from build123d import *

# Parameters (mm, degrees)
F0_R     = 25.4
F1_DEPTH = 12.7
F2_R     = 12.7
F3_DEPTH = 25.4
F4_R     = 2.54
F4_R_2   = 6.35
F5_DEPTH = 25.4


with BuildPart() as f1:
    # F0 (on Top) → F1 (new body)
    with BuildSketch(Plane.XY):
        Circle(F0_R)
    extrude(amount=F1_DEPTH)

    # F2 (on Top) → F3 (join)
    with BuildSketch(Plane.XY):
        Circle(F2_R)
    extrude(amount=F3_DEPTH)

    # F4 (on Top) → F5 (cut)
    with BuildSketch(Plane.XY):
        with Locations((0, 19.05)):
            Circle(F4_R)
        with Locations((-19.05, 0)):
            Circle(F4_R)
        with Locations((0, -19.05)):
            Circle(F4_R)
        with Locations((19.05, 0)):
            Circle(F4_R)
        Circle(F4_R_2)
    extrude(amount=F5_DEPTH, mode=Mode.SUBTRACT)


solid = f1.part
Source: CAD feature listing. Evaluate the final solid. Frame: model axes, mm. Give positions to 0.01 mm unless a question says otherwise; leave off trailing zeros. Write each loop counter-clockwise with the first axis right and the second up, starting at its lowest first coordinate (ties: lowest second). Pieces come first, ordered by that corner, then holes. Notation, with made-up numbers: M -11,25 L 8,25 A33 cw 8,53 Z; hole C 33.5,12 d2. An arc over 180 degrees is marked long. Return JSON: item names as keys, results as strings. Group by question number.
1) Cut plane D-D, the plane z = 20.75. Output: boundary loops of the cut face in (x, y), plus the area to 3 significant figures.
2) Cut plane C-C, the plane x = -19.05. Output: boundary loops of the cut face in (y, z), plus the area to 3 significant figures.
3) Pull-direction query (Y, two-part tool) for faces 1 (the face through (-0.33, -16.53, 6.26)), 2 (the face through (-12, -5, 12.7)), 3 (the face through (-2.75, -12.4, 18.96)); classes: pulls with the +Y half, pulls with the -Y half, needs draft (parallel to the pull), parting line crosses it, or undercut.
4) Pin query (flat end, axial travel): P1, Ø3, axis at y = -1.5, z = 8.5, coming from the +X side; P2, Ø7.5, axis at x = 0, y = 0, coming from the -Z side; P3, Ø1.5, axis at y = 8, z = 11, coming from the -X side; P4, Ø5, axis at x = 4, z = 13.5, coming from the -Y side. Return the tip coordinate at first contact, or that it passes through.
5) Cut plane A-A, the plane x = 0. Output: boundary loops of the cut face in (y, z).
6) Material intervals for line 1 along Y through (x, z) = (0, 9); line 2 along Z through (x, y) = (-9, -17.5); line 3 along X through (y, z) = (19.05, 10.25), sorted ascending. Write a range as [from, to].
7) Cut plane B-B, the plane y = 5. Output: boundary loops of the cut face in (x, z).
Recorded:
{
 "1": {"outline": "C 0,0 d25.4; hole C 0,0 d12.7", "area": "380 mm²"},
 "2": {"outline": "M -16.8,0 L -2.54,0 L -2.54,12.7 L -16.8,12.7 Z; M 2.54,0 L 16.8,0 L 16.8,12.7 L 2.54,12.7 Z", "area": "362 mm²"},
 "3": {"face 1": "undercut", "face 2": "needs draft", "face 3": "parting line crosses it"},
 "4": {"P1": "stops at x = 25.4", "P2": "passes through", "P3": "stops at x = -24.34", "P4": "stops at y = -25.35"},
 "5": {"outline": "M -25.4,0 L -21.59,0 L -21.59,12.7 L -25.4,12.7 Z; M -16.51,0 L -6.35,0 L -6.35,25.4 L -12.7,25.4 L -12.7,12.7 L -16.51,12.7 Z; M 6.35,0 L 16.51,0 L 16.51,12.7 L 12.7,12.7 L 12.7,25.4 L 6.35,25.4 Z; M 21.59,0 L 25.4,0 L 25.4,12.7 L 21.59,12.7 Z"},
 "6": {"line 1": "y = [-25.4, -21.59], [-16.51, -6.35], [6.35, 16.51], [21.59, 25.4]", "line 2": "z = [0, 12.7]", "line 3": "x = [-16.8, -2.54], [2.54, 16.8]"},
 "7": {"outline": "M -24.9,0 L -3.91,0 L -3.91,25.4 L -11.67,25.4 L -11.67,12.7 L -24.9,12.7 Z; M 3.91,0 L 24.9,0 L 24.9,12.7 L 11.67,12.7 L 11.67,25.4 L 3.91,25.4 Z"}
}
